Geometry check sheet. Reference: drawing and pictorial views, mm from the part's lowest x, y, z. Give positions to 0.01 mm unless a question says otherwise; leave off trailing zeros. Order: outer loops, then holes, each group sorted by start corner. A loop starts at its lowest first (then second) coordinate and runs counter-clockwise, first axis right, second up.
Item 1: Gauge pin test, flat ends, axial feed: P1, Ø1, axis at y = 8, z = 2, coming from the -X side; P2, Ø1.5, axis at y = 13.5, z = 2, coming from the -X side; P3, Ø3, axis at x = 1, y = 19.5, coming from the -Z side; P4, Ø2, axis at x = 4, z = 4, coming from the +Y side. Record the tip position at first contact, or that the pin passes through.
Item 2: Material ranges on line 1 along Z through (x, y) = (4, 21.7); line 2 along Z through (x, y) = (4, 12); line 3 along Y through (x, z) = (5.25, 1.5), recorded low to high.
Item 3: Sectioned sample at C-C on y = 18.5. Record the boundary of the cut face in (x, z), and give its area (3 significant figures).
Item 4: Sectioned sample at D-D on x = 2.5. Record the boundary of the cut face in (y, z).
Item 5: Sectioned sample at B-B on x = 4. Record the boundary of the cut face in (y, z), and give its area (3 significant figures).
Item 6: Sectioned sample at A-A on z = 4. Record the boundary of the cut face in (x, y).
Item 7: Release check for a two-part mould opening along X. For the marked faces 1, 2 and 3 record: released by +X, released by -X, zero draft, split by the parting line, or undercut.
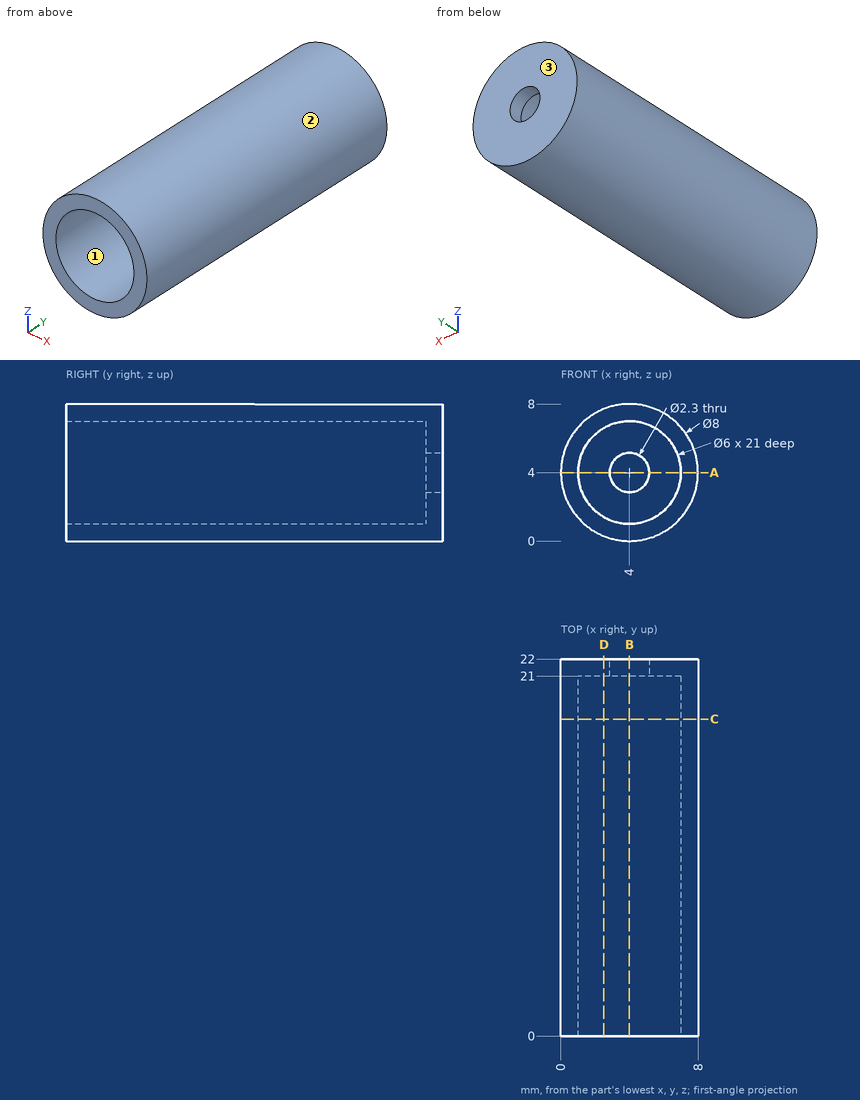
Report:
1. P1: stops at x = 0.29
1. P2: stops at x = 0.2
1. P3: stops at z = 0.29
1. P4: passes through
2. line 1: z = 0 to 2.85, 5.15 to 8
2. line 2: z = 0 to 1, 7 to 8
2. line 3: y = 21 to 22
3. outline: circle Ø8 at (4, 4); hole circle Ø6 at (4, 4)
3. area: 22.0 mm2
4. outline: (0, 0.29) - (22, 0.29) - (22, 7.71) - (0, 7.71) - (0, 6.6) - (21, 6.6) - (21, 1.4) - (0, 1.4) - close
5. outline: (0, 0) - (22, 0) - (22, 2.85) - (21, 2.85) - (21, 1) - (0, 1) - close; (0, 7) - (21, 7) - (21, 5.15) - (22, 5.15) - (22, 8) - (0, 8) - close
5. area: 47.7 mm2
6. outline: (0, 0) - (1, 0) - (1, 21) - (2.85, 21) - (2.85, 22) - (0, 22) - close; (5.15, 21) - (7, 21) - (7, 0) - (8, 0) - (8, 22) - (5.15, 22) - close
7. face 1: undercut
7. face 2: split by the parting line
7. face 3: zero draft
